Model file for the job. Use its own axes, mm. Face numbers are marked on the shaded views. A direction names the side the tool comes from. Round coordinates to 2 decimals unless told otherwise and drop trailing zeros. Loops run counter-clockwise (first coordinate to the right, second up) from the corner with the lowest first, then second, coordinate; pieces in that order, holes last. Notation, with made-up numbers: (-12.75, 79.25) - (-3.75, 79.25) arc R5 ccw to (-3.75, 84.25) - close; hole circle Ø3 at (18.5, -18). An arc over 180 degrees is marked (long way). Answer as a JSON object with one key per item and string values.
from build123d import *

# Parameters (mm, degrees)
SKETCH1_W                = 63.5
SKETCH1_H                = 38.1
BASE_DEPTH               = 3.175
SKETCH3_W                = 6.35
SKETCH3_H                = 38.1
ROD_HOLDER_DEPTH         = 15.875
SKETCH4_R                = 1.6
ROD_HOLE_DEPTH           = 87.660634806
SKETCH7_R                = 5.25
GEARPINHOLE_10_5MM_DEPTH = 81.572467382
SKETCH9_W                = 76.2
SKETCH9_H                = 3.175
BOSS_EXTRUDE1_DEPTH      = 15.875
SKETCH11_W               = 8.195400186
SKETCH11_H               = 19.05
BOSS_EXTRUDE2_DEPTH      = 15.2
SKETCH20_W               = 1
SKETCH20_H               = 19.05
BOSS_EXTRUDE7_DEPTH      = 15.2
SKETCH12_R               = 1.5
CUT_EXTRUDE1_DEPTH       = 8.89
BOSS_EXTRUDE3_DEPTH      = 15.2
SKETCH14_R               = 1.75
CUT_EXTRUDE2_DEPTH       = 6.858
SKETCH15_W               = 63.5
SKETCH15_H               = 0.79375
CUT_EXTRUDE3_DEPTH       = 12.7
SKETCH16_W               = 9.195400186
SKETCH16_H               = 2.2
SKETCH16_W_2             = 8.195400186
CUT_EXTRUDE4_DEPTH       = 4
BOSS_EXTRUDE4_DEPTH      = 1.5875
BOSS_EXTRUDE4_DEPTH_BACK = 1.5875
BOSS_EXTRUDE4_START      = -22.225
SKETCH18_R               = 5
BOSS_EXTRUDE5_DEPTH      = 6.35
BOSS_EXTRUDE6_DEPTH      = 3.175
FILLET1_R                = 1.27
FILLET2_R                = 1.27
SKETCH21_R               = 5
BOSS_EXTRUDE8_DEPTH      = 6.35


with BuildPart() as part:
    # Sketch1 → Base (new body)
    with BuildSketch(Plane(origin=(0, 0, 0), x_dir=(1, 0, 0), z_dir=(0, 1, 0))):
        with Locations((31.75, 19.05)):
            Rectangle(SKETCH1_W, SKETCH1_H)
    extrude(amount=BASE_DEPTH)

    # Sketch3 → Rod Holder (add)
    with BuildSketch(Plane(origin=(0, 0, 0), x_dir=(1, 0, 0), z_dir=(0, 1, 0))):
        with Locations((-3.175, 19.05)):
            Rectangle(SKETCH3_W, SKETCH3_H)
        with Locations((66.675, 19.05)):
            Rectangle(SKETCH3_W, SKETCH3_H)
    extrude(amount=ROD_HOLDER_DEPTH)

    # Sketch4 → Rod Hole (cut, through all)
    with BuildSketch(Plane(origin=(69.85, 0, 0), x_dir=(0, 0, -1), z_dir=(1, 0, 0))):
        with Locations((6.35, 12.7)):
            Circle(SKETCH4_R)
        with Locations((31.75, 12.7)):
            Circle(SKETCH4_R)
    extrude(amount=-ROD_HOLE_DEPTH, mode=Mode.SUBTRACT)

    # Sketch7 → GearPinHole_10.5mm (cut, through all)
    with BuildSketch(Plane(origin=(0, 3.175, 0), x_dir=(1, 0, 0), z_dir=(0, 1, 0))):
        with Locations(Location((31.75, 19.05, 0), (0, 0, 270))):
            Circle(SKETCH7_R)
    extrude(amount=-GEARPINHOLE_10_5MM_DEPTH, mode=Mode.SUBTRACT)

    # Sketch9 → Boss-Extrude1 (add)
    with BuildSketch(Plane.XZ):
        with Locations((31.75, 1.5875)):
            Rectangle(SKETCH9_W, SKETCH9_H)
        with Locations((31.75, -39.6875)):
            Rectangle(SKETCH9_W, SKETCH9_H)
    extrude(amount=-BOSS_EXTRUDE1_DEPTH)

    # Sketch11 → Boss-Extrude2 (add)
    with BuildSketch(Plane.XZ):
        with Locations((15.752300005, -19.05)):
            Rectangle(SKETCH11_W, SKETCH11_H)
        with Locations((65.752299907, -19.05)):
            Rectangle(SKETCH11_W, SKETCH11_H)
    extrude(amount=BOSS_EXTRUDE2_DEPTH)

    # Sketch20 → Boss-Extrude7 (add)
    with BuildSketch(Plane.XZ):
        with Locations((20.350000098, -19.05)):
            Rectangle(SKETCH20_W, SKETCH20_H)
    extrude(amount=BOSS_EXTRUDE7_DEPTH)

    # Sketch12 → Cut-Extrude1 (cut)
    with BuildSketch(Plane.XZ.offset(15.2)):
        with Locations(Location((17.75230014, -14.05, 0), (0, 0, 270))):
            Circle(SKETCH12_R)
        with Locations(Location((17.75230014, -24.05, 0), (0, 0, 270))):
            Circle(SKETCH12_R)
        with Locations(Location((65.752299962, -24.05, 0), (0, 0, 270))):
            Circle(SKETCH12_R)
        with Locations(Location((65.752299962, -14.05, 0), (0, 0, 270))):
            Circle(SKETCH12_R)
    extrude(amount=-CUT_EXTRUDE1_DEPTH, mode=Mode.SUBTRACT)

    # Sketch13 → Boss-Extrude3 (add)
    with BuildSketch(Plane.XZ):
        Polygon((11.654599912, -28.575), (16.734599912, -28.575), (16.734599912, -34.417), (64.77, -34.417), (64.77, -28.575), (69.85, -28.575), (69.85, -41.275), (11.654599912, -41.275), align=None)
    extrude(amount=BOSS_EXTRUDE3_DEPTH)

    # Sketch14 → Cut-Extrude2 (cut)
    with BuildSketch(Plane(origin=(0, 0, -41.275), x_dir=(-1, 0, 0), z_dir=(0, 0, -1))):
        with Locations((-53.752299956, -7.6)):
            Circle(SKETCH14_R)
        with Locations((-27.752299956, -7.6)):
            Circle(SKETCH14_R)
    extrude(amount=-CUT_EXTRUDE2_DEPTH, mode=Mode.SUBTRACT)

    # Sketch15 → Cut-Extrude3 (cut)
    with BuildSketch(Plane(origin=(0, 15.875, 0), x_dir=(1, 0, 0), z_dir=(0, 1, 0))):
        with Locations((31.75, 38.496875)):
            Rectangle(SKETCH15_W, SKETCH15_H)
        with Locations((31.75, -0.396875)):
            Rectangle(SKETCH15_W, SKETCH15_H)
    extrude(amount=-CUT_EXTRUDE3_DEPTH, mode=Mode.SUBTRACT)

    # Sketch16 → Cut-Extrude4 (cut)
    with BuildSketch(Plane.XZ.offset(15.2)):
        with Locations((16.252300005, -19.05)):
            Rectangle(SKETCH16_W, SKETCH16_H)
        with Locations((65.752299907, -19.05)):
            Rectangle(SKETCH16_W_2, SKETCH16_H)
    extrude(amount=-CUT_EXTRUDE4_DEPTH, mode=Mode.SUBTRACT)

    # Sketch17 → Boss-Extrude4 (add, two sides: drawn at the far end of the back side and taken through both)
    with BuildSketch(Plane(origin=(0, 0, -41.275), x_dir=(-1, 0, 0), z_dir=(0, 0, -1)).offset(BOSS_EXTRUDE4_START - BOSS_EXTRUDE4_DEPTH_BACK)):
        Polygon((-69.85, 0), (-82.55, 0), (-82.55, 25.4), (-79.375, 25.4), (-79.375, 3.175), (-69.85, 3.175), align=None)
    extrude(amount=BOSS_EXTRUDE4_DEPTH + BOSS_EXTRUDE4_DEPTH_BACK)

    # Sketch18 → Boss-Extrude5 (add)
    with BuildSketch(Plane(origin=(0, 25.4, 0), x_dir=(1, 0, 0), z_dir=(0, 1, 0))):
        with BuildLine():
            Line((82.55, 20.6375), (84.263823045, 20.6375))
            ThreePointArc((84.263823045, 20.6375), (96.05, 19.05), (84.263823045, 17.4625))
            Line((84.263823045, 17.4625), (82.55, 17.4625))
            Line((82.55, 17.4625), (82.55, 20.6375))
        make_face()
        with Locations(Location((90.05, 19.05, 0), (0, 0, 180))):
            Circle(SKETCH18_R, mode=Mode.SUBTRACT)
    extrude(amount=-BOSS_EXTRUDE5_DEPTH)

    # Sketch19 → Boss-Extrude6 (add)
    with BuildSketch(Plane(origin=(0, 0, -20.6375), x_dir=(-1, 0, 0), z_dir=(0, 0, -1))):
        Polygon((-79.375, 15.875), (-69.85, 6.35), (-69.85, 3.175), (-79.375, 12.7), align=None)
    extrude(amount=-BOSS_EXTRUDE6_DEPTH)

    # Fillet1
    fillet1_edges = [part.edges().sort_by_distance(p)[0] for p in [
        (82.55, 0, -19.05),
        (79.375, 3.175, -19.05),
        (79.375, 12.7, -19.05),
        (79.375, 15.875, -19.05),
        (69.85, 6.35, -19.05),
    ]]
    fillet(fillet1_edges, radius=FILLET1_R)

    # Fillet2
    # the kernel refuses this fillet: 1.27 mm, written as the material it adds along each edge
    with BuildSketch(Plane(origin=(69.85, 3.175, -17.4625), x_dir=(1, 0, 0), z_dir=(0, 0, -1))) as fillet2_piece_1:
        with BuildLine():
            CenterArc((FILLET2_R * 2.41421356237, -FILLET2_R), FILLET2_R, 90, 135)
            Line((FILLET2_R * 1.70710678119, -FILLET2_R * 1.70710678119), (0, 0))
            Line((0, 0), (FILLET2_R * 2.41421356237, 0))
        make_face()
    extrude(amount=3.175)

    # Sketch21 → Boss-Extrude8 (add)
    with BuildSketch(Plane(origin=(0, 25.4, 0), x_dir=(1, 0, 0), z_dir=(0, 1, 0))):
        with Locations((90.05, 19.05)):
            Circle(SKETCH21_R)
    extrude(amount=-BOSS_EXTRUDE8_DEPTH)

    # Sketch22 → Revolve1 (revolve)
    with BuildSketch(Plane.XY.offset(-19.05), mode=Mode.PRIVATE) as revolve1_sk:
        Polygon((90.05, 25.4), (90.05, 44.45), (96.05, 25.4), align=None)
    revolve(revolve1_sk.sketch.rotate(Axis((90.05, 25.4, -19.05), (0, 1, 0)), 90), axis=Axis((90.05, 25.4, -19.05), (0, 1, 0)))


solid = part.part
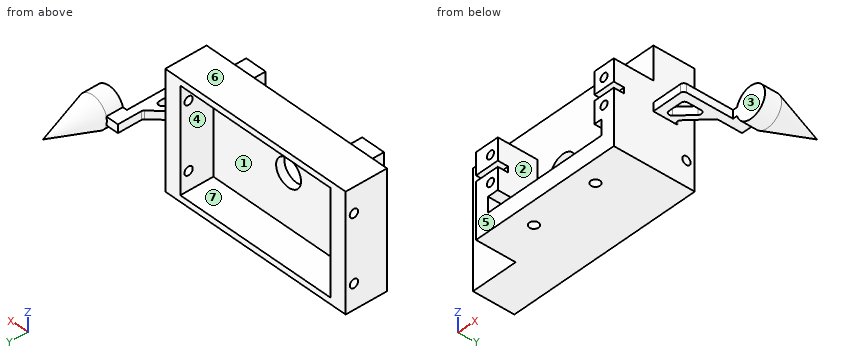
1) Slice it at C-C on x = 31.75. List the corners of the cut face in (y, z) (3 decimals), then the cut area to 3 significant figures.
Values follow:
{"outline": "(-15.2, -41.275) - (15.875, -41.275) - (15.875, -38.894) - (3.175, -38.894) - (3.175, -24.3) - (0, -24.3) - (0, -34.417) - (-15.2, -34.417) - close; (0, -13.8) - (3.175, -13.8) - (3.175, 0.794) - (15.875, 0.794) - (15.875, 3.175) - (0, 3.175) - close", "area": "273 mm²"}
2) Probe probe 1 along X at (y, z) = (-9.75, -14.05); probe 2 along X at (y, z) = (-8.5, -31); probe 3 along Z at (x, y) = (6.5, 7) (3 decimals). List the from-to ranges inside material, lowest first.
Values follow:
{"probe 1": "11.65 to 16.25, 19.25 to 20.85, 61.65 to 64.25, 67.25 to 69.85", "probe 2": "11.65 to 16.73, 64.77 to 69.85", "probe 3": "-41.275 to -38.894, 0.794 to 3.175"}
3) Drop flat-ended pins along their axis: P1, Ø1.6, axis at y = 22, z = -20, coming from the -X side (3 decimals); P2, Ø6, axis at y = -8, z = -24.5, coming from the +X side; P3, Ø5, axis at y = 23, z = -13, coming from the +X side. Give the stop position or say it passes through.
Values follow:
{"P1": "x = 79.375", "P2": "x = 69.85", "P3": "x = 94.89"}
4) Slice it at B-B on z = -31.75. List the corners of the cut face in (x, y) (3 decimals), then the cut area to 3 significant figures.
Values follow:
{"outline": "(-6.35, 0) - (11.655, 0) - (11.655, -15.2) - (16.735, -15.2) - (16.735, 0) - (64.77, 0) - (64.77, -15.2) - (69.85, -15.2) - (69.85, 11.1) - (63.5, 11.1) - (63.5, 3.175) - (0, 3.175) - (0, 11.1) - (-6.35, 11.1) - close; (-6.35, 14.3) - (0, 14.3) - (0, 15.875) - (-6.35, 15.875) - close; (63.5, 14.3) - (69.85, 14.3) - (69.85, 15.875) - (63.5, 15.875) - close", "area": "517 mm²"}
5) Tool access for the marked faces 1, 2 and 3: list every direction of +Z, -Z, +X, -X, +Y, -Y with a clear straight run to the whole face (end or side of a thin tool).
Values follow:
{"face 1": "+Y", "face 2": "+Z, -Y", "face 3": "+Z, -Z, +X, -Y"}
6) Slice it at D-D on z = -3.5. List the corners of the cut face in (x, y) (3 decimals).
Values follow:
{"outline": "(-6.35, 0) - (69.85, 0) - (69.85, 15.875) - (63.5, 15.875) - (63.5, 3.175) - (0, 3.175) - (0, 15.875) - (-6.35, 15.875) - close"}
7) Two-plate mould, pull along Z, no slides. Class the marked faces 4, 5, 6 and 7: pulls with the +Z half, pulls with the -Z half, needs draft (parallel to the pull), parting line crosses it, or undercut.
Values follow:
{"face 4": "undercut", "face 5": "needs draft", "face 6": "pulls with the +Z half", "face 7": "undercut"}
8) Slice it at A-A on y = -7.6. List the corners of the cut face in (x, z) (3 decimals), then the cut area to 3 significant figures.
Values follow:
{"outline": "(11.655, -41.275) - (26.002, -41.275) - (26.002, -34.417) - (16.735, -34.417) - (16.735, -28.575) - (20.85, -28.575) - (20.85, -9.525) - (11.655, -9.525) - close; (29.502, -41.275) - (52.002, -41.275) - (52.002, -34.417) - (29.502, -34.417) - close; (55.502, -41.275) - (69.85, -41.275) - (69.85, -9.525) - (61.655, -9.525) - (61.655, -28.575) - (64.77, -28.575) - (64.77, -34.417) - (55.502, -34.417) - close; hole circle Ø3 at (17.752, -24.05); hole circle Ø3 at (17.752, -14.05); hole circle Ø3 at (65.752, -24.05); hole circle Ø3 at (65.752, -14.05)", "area": "713 mm²"}
